Design review of the part shown in the three views and the two pictorial views. Dimensions are in mm from the part's minimum x, y and z. Give positions to 0.01 mm unless a question says otherwise; leave off trailing zeros. Loops run counter-clockwise (first coordinate to the right, second up) from the corner with the lowest first, then second, coordinate; pieces in that order, holes last. Notation, with made-up numbers: (-0.5, -1.75) - (24.5, -1.75) arc R17 cw to (24.5, 19.25) - close; hole circle Ø11 at (54.5, 31.25). An arc over 180 degrees is marked (long way). Return JSON: item names as keys, results as strings. Group by question number.
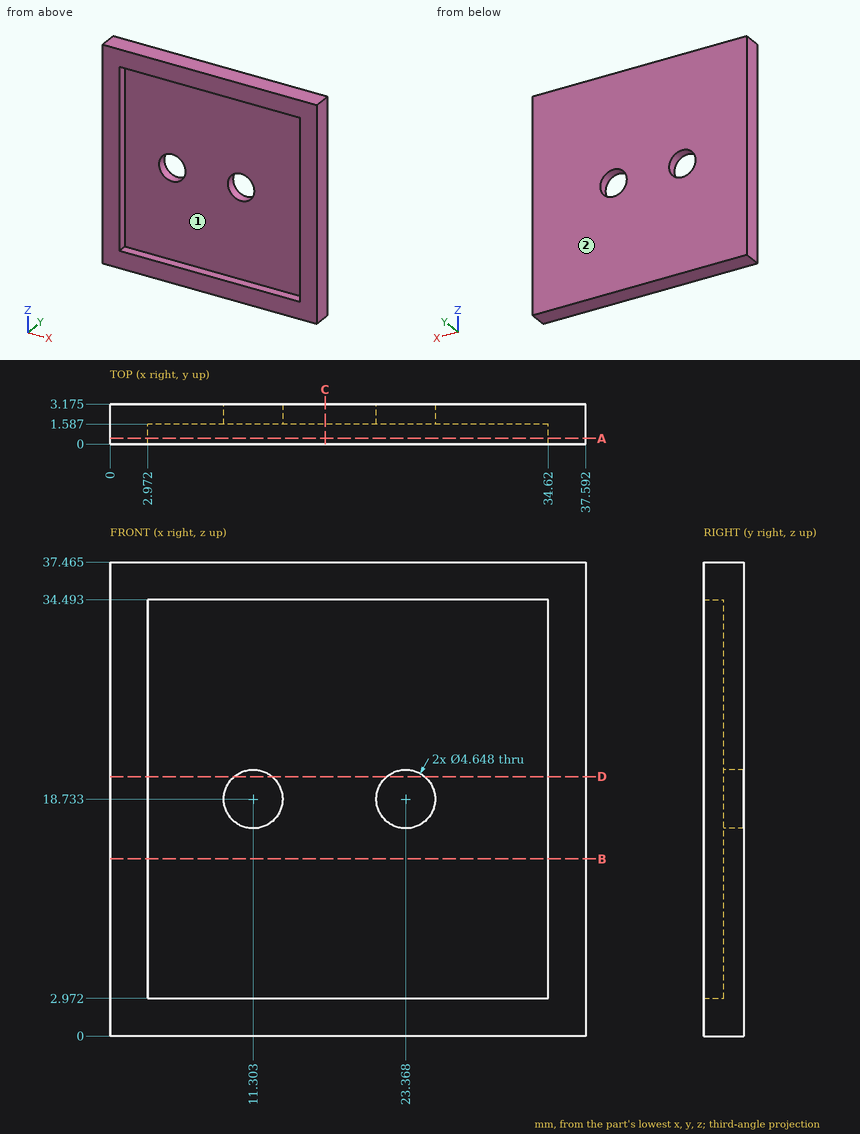
Item 1: For P1, Ø2, axis at x = 29, z = 23.5, coming from the -Y side; P2, Ø0.5, axis at x = 13.5, y = 1, coming from the -Z side; P3, Ø4, axis at x = 11.3, z = 18.73, coming from the +Y side, all flat-tipped, find the tip position at first contact; note any pin that passes through.
Item 2: Take a section at A-A (y = 0.45). State the section outline as (x, z) points (1 decimal), then the cut area to 3 significant figures.
Item 3: Take a section at B-B (z = 14). State the section outline as (x, y) points (1 decimal).
Item 4: Take a section at D-D (z = 20.5). State the section outline as (x, y) points (1 decimal).
Item 5: Take a section at C-C (x = 17). State the section outline as (y, z) points (1 decimal).
Item 6: Mouldability with a two-part tool opening along X and no side actions: class the marked faces 1 and 2 as +X half, -X half, draft (parallel to the pull), parting line (faces both ways), or undercut.
Item 7: For L1, parallel to X at y = 0.2, z = 28.5; L2, parallel to Z at x = 23.5, y = 2.85 (1 decimal); L3, parallel to Z at x = 23.5, y = 0.65 (1 decimal), list the stretches that pass through material, from the lowest coordinate up. Write a range as from..to.
Check sheet entries:
{
 "1": {"P1": "stops at y = 1.59", "P2": "stops at z = 0", "P3": "passes through"},
 "2": {"outline": "(0, 0) - (37.6, 0) - (37.6, 37.5) - (0, 37.5) - close; hole (3, 3) - (34.6, 3) - (34.6, 34.5) - (3, 34.5) - close", "area": "411 mm^2"},
 "3": {"outline": "(0, 0) - (3, 0) - (3, 1.6) - (34.6, 1.6) - (34.6, 0) - (37.6, 0) - (37.6, 3.2) - (0, 3.2) - close"},
 "4": {"outline": "(0, 0) - (3, 0) - (3, 1.6) - (9.8, 1.6) - (9.8, 3.2) - (0, 3.2) - close; (12.8, 1.6) - (21.9, 1.6) - (21.9, 3.2) - (12.8, 3.2) - close; (24.9, 1.6) - (34.6, 1.6) - (34.6, 0) - (37.6, 0) - (37.6, 3.2) - (24.9, 3.2) - close"},
 "5": {"outline": "(0, 0) - (3.2, 0) - (3.2, 37.5) - (0, 37.5) - (0, 34.5) - (1.6, 34.5) - (1.6, 3) - (0, 3) - close"},
 "6": {"face 1": "undercut", "face 2": "draft"},
 "7": {"L1": "x = 0..2.97, 34.62..37.59", "L2": "z = 0..16.4, 21.1..37.5", "L3": "z = 0..3, 34.5..37.5"}
}
